```python
from build123d import *

# Parameters (mm, degrees)
SKETCH1_R               = 1.6
BOSS_EXTRUDE1_DEPTH     = 2
BOSS_EXTRUDE2_START     = 7.41
BOSS_EXTRUDE2_DEPTH     = 7.41
CUT_EXTRUDE1_DEPTH      = 74.641853292
CUT_EXTRUDE1_DEPTH_BACK = 74.641853292
SKETCH3_R               = 1.6


with BuildPart() as part:
    # Sketch1 → Boss-Extrude1 (new body)
    with BuildSketch(Plane(origin=(0, 0, 0), x_dir=(1, 0, 0), z_dir=(0, 1, 0))):
        with BuildLine():
            Line((-5.70625, 0), (5.70625, 0))
            Line((5.70625, 0), (5.70625, -71.2))
            ThreePointArc((5.70625, -71.2), (3.584929656, -70.321320344), (2.70625, -68.2))
            Line((2.70625, -68.2), (-5.70625, -13.2))
            Line((-5.70625, -13.2), (-5.70625, 0))
        make_face()
        with Locations(Location((-2.70625, -3, 0), (0, 0, 270))):
            Circle(SKETCH1_R, mode=Mode.SUBTRACT)
        with Locations(Location((-2.70625, -10.5, 0), (0, 0, 270))):
            Circle(SKETCH1_R, mode=Mode.SUBTRACT)
    boss_extrude1 = extrude(amount=BOSS_EXTRUDE1_DEPTH)

    # Sketch2 → Boss-Extrude2 (add)
    with BuildSketch(Plane.XZ.offset(BOSS_EXTRUDE2_START)):
        with BuildLine():
            Line((5.70625, 71.2), (5.70625, 0))
            Line((5.70625, 0), (2.70625, 0))
            Line((2.70625, 0), (2.70625, 68.2))
            ThreePointArc((2.70625, 68.2), (3.584929656, 70.321320344), (5.70625, 71.2))
        make_face()
    boss_extrude2 = extrude(amount=-BOSS_EXTRUDE2_DEPTH)

    # Mirror6: Boss-Extrude2 across plane
    add(boss_extrude2.mirror(Plane(origin=(0, -7.41, 0), x_dir=(0, 0, 1), z_dir=(0, -1, 0))))

    # Mirror7: Boss-Extrude1 across plane
    add(boss_extrude1.mirror(Plane(origin=(0, -7.41, 0), x_dir=(0, 0, 1), z_dir=(0, -1, 0))))

    # Sketch3 → Cut-Extrude1 (cut, two sides: drawn at the far end of the back side and taken through both)
    with BuildSketch(Plane.ZY.offset(-2.70625).offset(-CUT_EXTRUDE1_DEPTH_BACK)):
        with Locations((24, -7.41)):
            Circle(SKETCH3_R)
        with Locations((12, -7.41)):
            Circle(SKETCH3_R)
    extrude(amount=CUT_EXTRUDE1_DEPTH + CUT_EXTRUDE1_DEPTH_BACK, mode=Mode.SUBTRACT)


solid = part.part
```
Model file for the job. Use its own axes, mm. A direction names the side the tool comes from. Give positions to 0.01 mm unless a question says otherwise; leave off trailing zeros. Order: outer loops, then holes, each group sorted by start corner. A loop starts at its lowest first (then second) coordinate and runs counter-clockwise, first axis right, second up.
1) Saw through at B-B, the plane z = 3. Write the cut outline in (x, y), then the cut area to 3 significant figures.
2) Saw through at A-A, the plane y = -7.41. Write the cut outline in (x, z).
3) Pin check, flat tips, straight feed: pin 1 (4 mm diameter, centred on y = -7.41, z = 24, fed in from +X); pin 2 (2 mm diameter, centred on x = 2.5, y = -7, fed in from +Z); pin 3 (4.5 mm diameter, centred on y = -7.5, z = 25.5, fed in from -X). Stop position of each tip, or through.
4) Saw through at D-D, the plane z = 11. Write the cut outline in (x, y), then the cut area to 3 significant figures.
5) Mould opens along X. For faces 3 (the cylindrical face through (-2.64, 0.99, 1.4)), 4 (the flat face through (4, -7, 0)), 5 (the flat face through (5.706, -7, 35)) say: +X half, -X half, draft (parallel to the pull), parting line (faces both ways), or undercut.
6) Saw through at C-C, the plane x = -0.5. Write the cut outline in (y, z), then the cut area to 3 significant figures.
7) Wall check: probe 1 along Y at (x, z) = (0.5, 29); probe 2 along Z at (x, y) = (4.5, -6.75); probe 3 along X at (y, z) = (-15.6, 3). Give the ranges that are in metal, low to high.
8) 3-axis set-ups, long thin cutter, end or side, ignore diameter. For faces 1 (the flat face through (0, -14.82, 26)), 2 (the cylindrical face through (-2.64, 0.99, 8.9)): which of +Z, -Z, +X, -X, +Y, -Y reach the whole face in a straight line?
Computed:
1. outline: (-5.71, -16.82) - (-4.31, -16.82) - (-4.31, -14.82) - (-5.71, -14.82) - close; (-5.71, 0) - (-4.31, 0) - (-4.31, 2) - (-5.71, 2) - close; (-1.11, -16.82) - (5.71, -16.82) - (5.71, 2) - (-1.11, 2) - (-1.11, 0) - (2.71, 0) - (2.71, -14.82) - (-1.11, -14.82) - close
1. area: 77.3 mm2
2. outline: (2.71, 0) - (5.71, 0) - (5.71, 10.4) - (2.71, 10.4) - close; (2.71, 13.6) - (5.71, 13.6) - (5.71, 22.4) - (2.71, 22.4) - close; (2.71, 25.6) - (5.71, 25.6) - (5.71, 71.2) arc R3 ccw to (2.71, 68.2) - close
3. pin 1: stops at x = 5.71
3. pin 2: stops at z = 70.23
3. pin 3: stops at x = 2.71
4. outline: (-5.71, -16.82) - (-4.23, -16.82) - (-4.23, -14.82) - (-5.71, -14.82) - close; (-5.71, 0) - (-4.23, 0) - (-4.23, 2) - (-5.71, 2) - close; (-1.19, -16.82) - (5.71, -16.82) - (5.71, -8.66) - (2.71, -8.66) - (2.71, -14.82) - (-1.19, -14.82) - close; (-1.19, 0) - (2.71, 0) - (2.71, -6.16) - (5.71, -6.16) - (5.71, 2) - (-1.19, 2) - close
4. area: 70.5 mm2
5. face 3: undercut
5. face 4: draft
5. face 5: +X half
6. outline: (-16.82, 0) - (-14.82, 0) - (-14.82, 47.24) - (-16.82, 47.24) - close; (0, 0) - (2, 0) - (2, 47.24) - (0, 47.24) - close
6. area: 189 mm2
7. probe 1: y = -16.82 to -14.82, 0 to 2
7. probe 2: z = 0 to 10.54, 13.46 to 22.54, 25.46 to 70.95
7. probe 3: x = -5.71 to -4.31, -1.11 to 5.71
8. face 1: +Z, -Z, -X
8. face 2: +Y, -Y
